Design review of the part built by this model. Coordinates are the model's own, in mm. Face numbers are marked on the shaded views. A direction names the side the tool comes from. Coordinates: 2 decimals unless noted, no trailing zeros. Write each loop counter-clockwise with the first axis right and the second up, starting at its lowest first coordinate (ties: lowest second). Pieces come first, ordered by that corner, then holes. Notation, with made-up numbers: M -5.5,46 L 18.5,46 A7 ccw 18.5,54 Z; hole C 52,-8 d8. An arc over 180 degrees is marked long. Return JSON: item names as keys, results as strings. Group by question number.
Autodesk Inventor part; units mm, degrees
ref_plane "Work Plane5" through (-25, 0, -21) normal (-1, 0, 0) x (0, 0, 1)
ref_plane "Work Plane4" through (25, 0, 21) normal (1, 0, 0) x (0, 0, -1)
ref_plane "Work Plane6" through (-25, 0, -21) normal (-1, 0, 0) x (0, 0, 1)
sketch "Sketch1" plane through (0, 0, 0) normal (0, 1, 0) x (-1, 0, 0)
  line L0 (21, 21) -> (-21, 21)
  line L1 (-21, 21) -> (-21, -21)
  line L2 (-21, -21) -> (21, -21)
  line L3 (21, -21) -> (21, 21)
  line L4 (21, 21) -> (-21, -21) construction
  line L5 (-21, 21) -> (21, -21) construction
  point P0 (0, 0)
  dimension "d0" = 42
  dimension "d1" = 42
extrude "Extrusion1" add sketch "Sketch1" along normal blind 6.5
sketch "Sketch2" plane through (0, 6.5, 0) normal (0, 1, 0) x (1, 0, 0)
  line L0 (-12, -12) -> (12, -12)
  line L1 (12, -12) -> (12, 12)
  line L2 (12, 12) -> (-12, 12)
  line L3 (-12, 12) -> (-12, -12)
  line L4 (-12, -12) -> (12, 12) construction
  line L5 (12, -12) -> (-12, 12) construction
  point P0 (0, 0)
  dimension "d4" = 24
  dimension "d5" = 24
extrude "Extrusion2" cut sketch "Sketch2" against normal blind 4.5
sketch "Sketch3" plane through (0, 2, 0) normal (0, 1, 0) x (1, 0, 0)
  line L0 (-10.5, -6) -> (-3.5, -6)
  line L1 (-3.5, -6) -> (-3.5, 6)
  line L2 (-3.5, 6) -> (-10.5, 6)
  line L3 (-10.5, 6) -> (-10.5, -6)
  line L4 (-10.5, -6) -> (-3.5, 6) construction
  line L5 (-3.5, -6) -> (-10.5, 6) construction
  line L6 (-12, -12) -> (-12, 12)
  line L7 (3.5, -6) -> (10.5, -6)
  line L8 (10.5, -6) -> (10.5, 6)
  line L9 (10.5, 6) -> (3.5, 6)
  line L10 (3.5, 6) -> (3.5, -6)
  line L11 (3.5, -6) -> (10.5, 6) construction
  line L12 (10.5, -6) -> (3.5, 6) construction
  line L13 (12, 12) -> (12, -12)
  point P0 (0, 0)
  point P1 (-7, 0)
  point P2 (-7, 0)
  point P3 (7, 0)
  point P4 (7, 0)
  dimension "d8" = 7
  dimension "d9" = 12
  dimension "d10" = 1.5
  dimension "d11" = 7
  dimension "d12" = 1.5
  dimension "d13" = 12
extrude "Extrusion3" cut sketch "Sketch3" against normal blind 3.5
sketch "Sketch4" plane through (0, 2, 0) normal (0, 1, 0) x (1, 0, 0)
  line L0 (-12, -12) -> (-12, 12)
  line L1 (12, -12) -> (-12, -12)
  point P0 (0, 0)
  point P1 (-8, -8)
  point P2 (-8, 8)
  point P3 (8, 8)
  point P4 (8, -8)
  dimension "d16" = 16
  dimension "d17" = 16
  dimension "d18" = 4
  dimension "d19" = 4
hole "Hole1" at (-8, 2, 8) at (-8, 2, -8) at (8, 2, -8) at (8, 2, 8) direction (0, -1, 0) diameter 4 end through all
sketch "Sketch5" plane through (0, 6.5, 0) normal (0, 1, 0) x (1, 0, 0)
  line L0 (-21, -21) -> (21, -21)
  line L1 (-21, 21) -> (-21, -21)
  point P0 (0, 0)
  point P1 (-15.2, -15.2)
  point P2 (-15.2, 15.2)
  point P3 (15.2, 15.2)
  point P4 (15.2, -15.2)
  dimension "d27" = 30.4
  dimension "d28" = 30.4
  dimension "d29" = 5.8
  dimension "d30" = 5.8
hole "Hole2" at (-15.2, 6.5, 15.2) at (-15.2, 6.5, -15.2) at (15.2, 6.5, -15.2) at (15.2, 6.5, 15.2) direction (0, -1, 0) diameter 4 end through all
ref_plane "Work Plane5" through (-25, 0, -21) normal (-1, 0, 0) x (0, 0, 1)
sketch "Sketch9" plane through (-25, 0, -21) normal (-1, 0, 0) x (0, 0, 1)
  point P0 (21, 0)
ref_plane "Work Plane4" through (25, 0, 21) normal (1, 0, 0) x (0, 0, -1)
sketch "Sketch10" plane through (25, 0, 21) normal (1, 0, 0) x (0, 0, -1)
  line L0 (27, 2) -> (31, 2)
  line L1 (27, 2) -> (15, 2)
  line L2 (11, 2) -> (15, 2)
  line L3 (15, 2) -> (27, 2)
  line L4 (27, 2) -> (31, 2)
  line L5 (27, 2) -> (15, 2)
  line L6 (11, 2) -> (15, 2)
  line L7 (15, 2) -> (27, 2)
  line L8 (33, 2) -> (9, 2)
  line L9 (9, 2) -> (33, 2)
  line L10 (27, 2) -> (15, 2)
  line L11 (27, 2) -> (27, 0)
  line L12 (15, 2) -> (27, 2)
  line L13 (15, 2) -> (15, 0)
  line L14 (27, 0) -> (15, 0)
  point P0 (21, 0)
extrude "Extrusion7" cut sketch "Sketch10" against normal blind 15
ref_plane "Work Plane6" through (-25, 0, -21) normal (-1, 0, 0) x (0, 0, 1)
sketch "Sketch11" plane through (-25, 0, -21) normal (-1, 0, 0) x (0, 0, 1)
  line L0 (27, 2) -> (27, 0)
  line L1 (15, 2) -> (27, 2)
  line L2 (15, 2) -> (15, 0)
  line L3 (27, 0) -> (15, 0)
  point P0 (21, 0)
extrude "Extrusion8" cut sketch "Sketch11" against normal blind 15
ref_plane "Work Plane7" through (-25, 0, 6) normal (-1, 0, 0) x (0, 0, 1)
ref_plane "Work Plane8" through (-25, 0, 6) normal (-1, 0, 0) x (0, 0, 1)
ref_plane "Work Plane9" through (-25, 2, -6) normal (0, -1, 0) x (1, 0, 0)
sketch "Sketch16" plane through (-25, 2, -6) normal (0, -1, 0) x (1, 0, 0)
  line L0 (13, 12) -> (13, 0)
  line L1 (4, 12) -> (13, 12)
  line L2 (4, 0) -> (13, 0)
  line L3 (37, 0) -> (37, 12)
  line L4 (50, 0) -> (37, 0)
  line L5 (50, 12) -> (50, 0)
  line L6 (50, 12) -> (37, 12)
  line L7 (4, 0) -> (4, 12)
  point P0 (25, 6)
extrude "Extrusion11" cut sketch "Sketch16" against normal blind 2
ref_plane "Work Plane10" through (-21, 6.5, 21) normal (1, 0, 0) x (0, 0, -1)
ref_plane "Work Plane11" through (-25, 0, 6) normal (-1, 0, 0) x (0, 0, 1)
fillet "Fillet4" radius 2 4 edges at (21, 0, -13.5) (21, 0, 13.5) (0, 0, -21) (0, 0, 21)
ref_plane "Work Plane12" through (-21.8, 6.5, 21) normal (1, 0, 0) x (0, 0, -1)
sketch "Sketch21" plane through (0, 0, 0) normal (0, -1, 0) x (1, 0, 0)
  circle A0 centre (8, 8) radius 2
  circle A1 centre (8, -8) radius 2
  circle A2 centre (-8, -8) radius 2
  circle A3 centre (-8, 8) radius 2
  circle A4 centre (-8, 8) radius 2
  line L0 (-10, 8) -> (-6, 8)
  line L1 (-6, 8) -> (-6, -8)
  line L2 (-6, -8) -> (-10, -8)
  line L3 (-10, -8) -> (-10, 8)
  line L4 (6, 8) -> (10, 8)
  line L5 (10, 8) -> (10, -8)
  line L6 (10, -8) -> (6, -8)
  line L7 (6, -8) -> (6, 8)
  point P0 (0, 0)
  point P1 (8, 6)
  point P2 (8, -6)
  point P3 (-8, -6)
  point P4 (-8, 6)
  point P5 (10, 8)
  point P6 (-6, 8)
extrude "Extrusion16" cut sketch "Sketch21" against normal blind 3 contours L5 A1 L7 A0 | A2 L3 A3 L1
properties part number "encoder_cover"
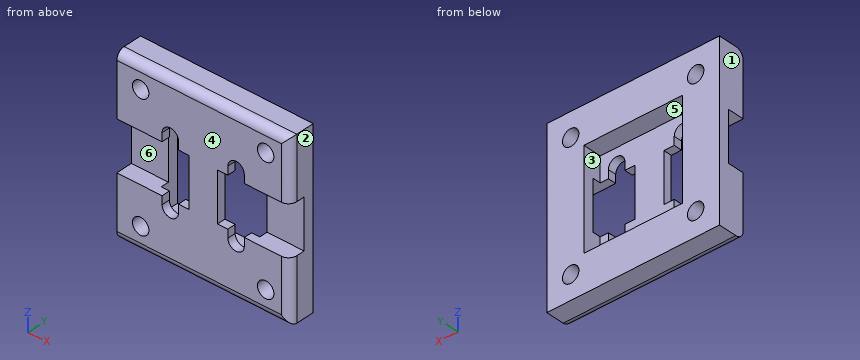
Item 1: Add section C-C (z = -2). Write out the cut boundary in (x, y).
Item 2: For pin 1 (0.6 mm diameter, centred on y = 1, z = 2, fed in from -X); pin 2 (7 mm diameter, centred on x = -17, z = 0.5, fed in from -Y); pin 3 (1 mm diameter, centred on x = -4.5, y = 1, fed in from -Z), all flat-tipped, find the tip position at first contact; note any pin that passes through.
Item 3: Add section D-D (y = 6). Write out the cut boundary in (x, z), plus the area to 3 significant figures.
Item 4: For line 1 (Z direction, x = -15.2, y = 4.75); line 2 (Z direction, x = -15.2, y = 2.75), list the stretches that pass through material, from the lowest coordinate up.
Item 5: The part is to be moulded in two halves that separate along X. For the marked faces 1, 2 and 3, say which applies: pulls with the +X half, pulls with the -X half, needs draft (parallel to the pull), parting line crosses it, or undercut.
Item 6: Add section B-B (x = -8). Write out the cut boundary in (y, z), plus the area to 3 significant figures.
Item 7: Machinability: for the marked faces 4, 5 and 6, which of the approach directions +Z, -Z, +X, -X, +Y, -Y give a long, thin tool a straight path to every point of the face, cutting with its end or side? Answer none if there is none.
Item 8: Add section A-A (y = 2.75). Write out the cut boundary in (x, z).
Geometry check:
{
 "1": {"outline": "M -21,4 L -12,4 L -12,6.5 L -21,6.5 Z; M -3.5,0 L 3.5,0 L 3.5,2 L -3.5,2 Z; M 12,4 L 21,4 L 21,6.5 L 12,6.5 Z"},
 "2": {"pin 1": "x = -3.5", "pin 2": "y = 4", "pin 3": "z = -20.94"},
 "3": {"outline": "M -21,-21 L 21,-21 L 21,21 L -21,21 Z; hole C -15.2,-15.2 d4; hole C -15.2,15.2 d4; hole M -12,-12 L 12,-12 L 12,12 L -12,12 Z; hole C 15.2,-15.2 d4; hole C 15.2,15.2 d4", "area": "1,140 mm^2"},
 "4": {"line 1": "-21 to -17.2, -13.2 to 13.2, 17.2 to 21", "line 2": "-21 to -17.2, -13.2 to -6, 6 to 13.2, 17.2 to 21"},
 "5": {"face 1": "pulls with the -X half", "face 2": "pulls with the +X half", "face 3": "undercut"},
 "6": {"outline": "M 0,-19 A2 ccw 2,-21 L 6.5,-21 L 6.5,-12 L 2,-12 L 2,-10 L 0,-10 Z; M 0,10 L 2,10 L 2,12 L 6.5,12 L 6.5,21 L 2,21 A2 ccw 0,19 Z", "area": "123 mm^2"},
 "7": {"face 4": "+Z, -Z, +X, -X, -Y", "face 5": "+Y", "face 6": "+X, -X, -Y"},
 "8": {"outline": "M -21,-21 L 21,-21 L 21,-6 L 12,-6 L 12,-12 L -12,-12 L -12,-6 L -21,-6 Z; M -21,6 L -12,6 L -12,12 L 12,12 L 12,6 L 21,6 L 21,21 L -21,21 Z; hole C -15.2,-15.2 d4; hole C -15.2,15.2 d4; hole C 15.2,-15.2 d4; hole C 15.2,15.2 d4"}
}
